Design review of the part built by this model. Coordinates are the model's own, in mm. A direction names the side the tool comes from. Give positions to 0.01 mm unless a question says otherwise; leave off trailing zeros. Order: outer loops, then holes, each group sorted by start corner. A loop starts at its lowest first (then second) coordinate and runs counter-clockwise, first axis right, second up.
```python
from build123d import *

# Parameters (mm, degrees)
F1_DEPTH = 25.4
F2_SIZE  = 5.08
F3_SIZE  = 5.08
F4_DEPTH = 25.4


with BuildPart() as f1:
    # F0 (on Top) → F1 (new body)
    with BuildSketch(Plane.XY):
        Polygon((-96.55295, 82.698783), (-135.158697, 19.198783), (68.041303, 19.198783), (36.314912, 82.698783), align=None)
        Polygon((-107.044348, 30.241039), (-113.656216, 30.241039), (-118.00166, 30.241039), (-93.268513, 70.743374), (-86.106063, 70.743374), (-79.70608, 70.743374), (-73.083729, 70.743374), (-48.325919, 70.743374), (-41.849952, 70.743374), (-35.128757, 70.743374), (-59.245978, 30.241039), (-66.7454, 30.241039), (-72.049234, 30.241039), (-78.653234, 30.241039), align=None, mode=Mode.SUBTRACT)
    extrude(amount=F1_DEPTH)

    # F2
    f2_edges = [f1.edges().sort_by_distance(p)[0] for p in [
        (-30.119019, 82.698783, 25.4),
        (-115.855824, 50.948783, 25.4),
        (52.178107, 50.948783, 25.4),
    ]]
    chamfer(f2_edges, length=F2_SIZE)

    # F3
    f3_edges = [f1.edges().sort_by_distance(p)[0] for p in [
        (-33.425499, 19.198783, 25.4),
    ]]
    chamfer(f3_edges, length=F3_SIZE)

    # F0 (on Top) → F4 (join)
    with BuildSketch(Plane.XY):
        Polygon((-72.049234, 30.241039), (-93.047231, 64.139374), (-113.656216, 30.241039), (-107.044348, 30.241039), (-92.57324, 57.535374), (-78.653234, 30.241039), align=None)
    extrude(amount=F4_DEPTH)


solid = f1.part
```
1. For pin 1 (8 mm diameter, centred on y = 50, z = 7.5, fed in from -X); pin 2 (8 mm diameter, centred on y = 42, z = 6, fed in from +X); pin 3 (3 mm diameter, centred on y = 53.5, z = 10.5, fed in from +X), all flat-tipped, find the tip position at first contact; note any pin that passes through.
Recorded:
pin 1: stops at x = -118.86
pin 2: stops at x = 58.65
pin 3: stops at x = 51.65
2. For line 1 along Y through (x, z) = (-60, 14.5); line 2 along X through (y, z) = (48.5, 24); line 3 along Y through (x, z) = (-99, 7), list the stretches that pass through material, from the lowest coordinate up.
Recorded:
line 1: y = 19.2 to 30.24, 70.74 to 82.7
line 2: x = -113.04 to -106.85, -102.56 to -97.36, -87.97 to -83.36, -48.37 to 49.29
line 3: y = 19.2 to 30.24, 45.41 to 54.35, 61.36 to 78.67
3. Take a section at D-D (y = 67.5). State the section outline as (x, z) points, then the cut area to 3 significant figures.
Recorded:
outline: (-105.79, 0) - (-95.25, 0) - (-95.25, 25.4) - (-99.85, 25.4) - (-105.79, 20.32) - close; (-37.06, 0) - (43.91, 0) - (43.91, 20.32) - (38.23, 25.4) - (-37.06, 25.4) - close
area: 2,290 mm2
4. Take a section at C-C (x = -47). State the section outline as (y, z) points, then the cut area to 3 significant figures.
Recorded:
outline: (19.2, 0) - (50.81, 0) - (50.81, 25.4) - (24.28, 25.4) - (19.2, 20.32) - close; (70.74, 0) - (82.7, 0) - (82.7, 20.32) - (77.62, 25.4) - (70.74, 25.4) - close
area: 1,080 mm2
5. Draft analysis for pull direction X (two halves, no side actions). For faces 1 (the face through (-116, 30.241, 13)), 2 (the face through (-105.808, 50.209, 12.522)), 3 (the face through (-12, 51, 0)), 4 (the face through (50.096, 49.353, 22.896)), state which applies: pulls with the +X half, pulls with the -X half, needs draft (parallel to the pull), parting line crosses it, or undercut.
Recorded:
face 1: undercut
face 2: undercut
face 3: needs draft
face 4: pulls with the +X half
6. Take a section at A-A (z = 10.5). State the section outline as (x, y) points, then the cut area to 3 significant figures.
Recorded:
outline: (-135.16, 19.2) - (68.04, 19.2) - (36.31, 82.7) - (-96.55, 82.7) - close; hole (-118, 30.24) - (-113.66, 30.24) - (-93.05, 64.14) - (-72.05, 30.24) - (-59.25, 30.24) - (-35.13, 70.74) - (-93.27, 70.74) - close; hole (-107.04, 30.24) - (-78.65, 30.24) - (-92.57, 57.54) - close
area: 8,620 mm2
7. Machinability: for faces 5 (the face through (-34.981, 21.774, 22.896)), 6 (the face through (-66, 30.241, 13)), which of the approach directions +Z, -Z, +X, -X, +Y, -Y give a long, thin tool a straight path to every point of the face, cutting with its end or side? Answer none if there is none.
Recorded:
face 5: +Z, +X, -X, -Y
face 6: +Z, -Z
8. Take a section at B-B (y = 50). State the section outline as (x, z) points, then the cut area to 3 significant figures.
Recorded:
outline: (-116.43, 0) - (-105.94, 0) - (-105.94, 25.4) - (-110.49, 25.4) - (-116.43, 20.32) - close; (-101.64, 0) - (-96.57, 0) - (-96.57, 25.4) - (-101.64, 25.4) - close; (-88.73, 0) - (-84.29, 0) - (-84.29, 25.4) - (-88.73, 25.4) - close; (-47.48, 0) - (52.65, 0) - (52.65, 20.32) - (46.97, 25.4) - (-47.48, 25.4) - close
area: 3,020 mm2
